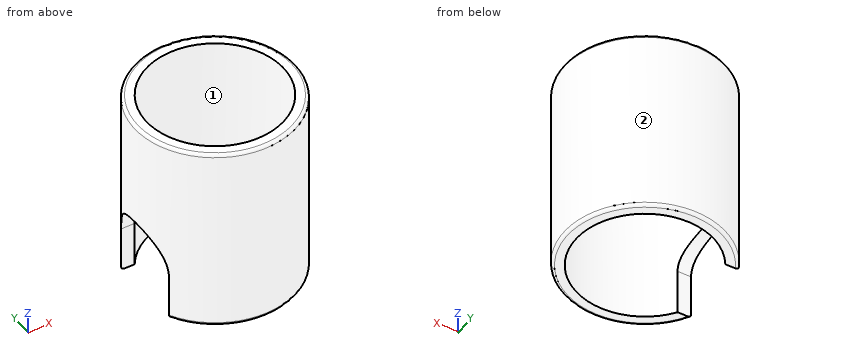
```python
from build123d import *

# Parameters (mm, degrees)
SKETCH_1_R          = 5.3
SKETCH_1_R_2        = 4.525
EXTRUDE_1_DEPTH     = 12.5
SKETCH_2_R          = 2.5
SKETCH_2_W          = 3.970430226
SKETCH_2_H          = 5
CUT_EXTRUDE_1_DEPTH = 12.5
FILLET_1_R          = 0.2


with BuildPart() as part:
    # 草图1 → 凸台-拉伸1 (new body)
    with BuildSketch(Plane.XY):
        Circle(SKETCH_1_R)
        Circle(SKETCH_1_R_2, mode=Mode.SUBTRACT)
    extrude(amount=EXTRUDE_1_DEPTH)

    # 草图2 → 切除-拉伸1 (cut)
    with BuildSketch(Plane(origin=(0, 0, 0), x_dir=(0, 0, -1), z_dir=(1, 0, 0))):
        with Locations((-3, 0)):
            Circle(SKETCH_2_R)
        with Locations((-1.014784887, 0)):
            Rectangle(SKETCH_2_W, SKETCH_2_H)
    extrude(amount=-CUT_EXTRUDE_1_DEPTH, mode=Mode.SUBTRACT)

    # 圆角1
    fillet_1_edges = [part.edges().sort_by_distance(p)[0] for p in [
        (1.288673453, 5.14094551, 0),
        (-5.3, 0, 12.5),
    ]]
    fillet(fillet_1_edges, radius=FILLET_1_R)


solid = part.part
```
Could you check a few things on this model? Use its own coordinates, in mm. Face numbers are marked on the shaded views. Round coordinates to 2 decimals unless told otherwise and drop trailing zeros. Loops run counter-clockwise (first coordinate to the right, second up) from the corner with the lowest first, then second, coordinate; pieces in that order, holes last. Notation, with made-up numbers: M -20,-15 L -3,-15 A35 ccw -3,18 Z; hole C 75,-3 d1. An arc over 180 degrees is marked long. Write item = value, one per line.
1. I want a section at A-A, the plane x = 0. Write out the boundary of the cut face in (y, z) (3 decimals), and give its area (3 significant figures).
Results below:
outline = M -5.3,0.2 A0.2 ccw -5.1,0 L -4.525,0 L -4.525,12.5 L -5.1,12.5 A0.2 ccw -5.3,12.3 Z; M 4.525,0 L 5.1,0 A0.2 ccw 5.3,0.2 L 5.3,12.3 A0.2 ccw 5.1,12.5 L 4.525,12.5 Z
area = 19.3 mm²
2. I want a section at C-C, the plane z = 1.5. Write out the boundary of the cut face in (x, y) (3 decimals), and give its area (3 significant figures).
Results below:
outline = M -4.673,-2.5 A5.3 ccw long -4.673,2.5 L -3.772,2.5 A4.525 cw long -3.772,-2.5 Z
area = 19.9 mm²
3. I want a section at B-B, the plane z = 8. Write out the boundary of the cut face in (x, y) (3 decimals).
Results below:
outline = C 0,0 d10.6; hole C 0,0 d9.05
4. Thinking about a two-plate mould opening in Y: for the marked faces 1 and 2, which applies, +Y half, -Y half, draft (parallel to the pull), parting line (faces both ways), or undercut?
Results below:
face_1 = undercut
face_2 = parting line
5. I need wall thicknesses on probe 1 along Y at (x, z) = (0, 4.25) (3 decimals); probe 2 along X at (y, z) = (3, 4.5). Which ranges of each line are inside material? Lowest first, please.
Results below:
probe_1 = -5.3 to -4.525, 4.525 to 5.3
probe_2 = -4.37 to -3.39, 3.39 to 4.37
6. Will these pins go through, and if not, where does the flat tip stop? P1, Ø1, axis at y = -3, z = 2.5, coming from the +X side; P2, Ø3, axis at y = 0.5, z = 4.5, coming from the -X side; P3, Ø1, axis at x = -1.5, z = 11, coming from the -Y side; P4, Ø2, axis at x = 3, z = 2, coming from the +Y side.
Results below:
P1 = 4.67
P2 = -5.3
P3 = -5.2
P4 = 4.91
